Geometry: final body of the model. Coordinates: model frame, mm. Face numbers are marked on the shaded views. A direction names the side the tool comes from. Coordinates: 2 decimals unless noted, no trailing zeros. Order: outer loops, then holes, each group sorted by start corner. A loop starts at its lowest first (then second) coordinate and runs counter-clockwise, first axis right, second up. Notation, with made-up numbers: M -16,-12 L 14,-12 A29 cw 14,17 Z; hole C 39.5,-13 d11. An arc over 180 degrees is marked long. Write item = value, one per line.
from build123d import *

# Parameters (mm, degrees)
EXTRUDE006_DEPTH = 7
EXTRUDE002_DEPTH = 15


with BuildPart() as extrude006:
    # Sketch007 → Extrude006 (new body)
    with BuildSketch(Plane(origin=(0, 20, 0), x_dir=(-1, 0, 0), z_dir=(0, 1, 0))):
        Polygon((-90, 0), (-69.999121, 80.000221), (-19.999121, 80.000221), (0, 0), align=None)
    extrude(amount=EXTRUDE006_DEPTH)


with BuildPart() as fusion:
    # Sketch003 → Extrude002 (new body)
    with BuildSketch(Plane.XZ):
        Polygon((6.519191, 4.955519), (24.519191, 74.72189), (66.519191, 74.72189), (84.519191, 4.955519), align=None)
    extrude(amount=EXTRUDE002_DEPTH)


with BuildPart() as fusion_1:
    # Extrude002 placement: moved
    add(fusion.part.moved(Location((0, 26, 0))))

    # Fusion: union Extrude006
    add(extrude006.part)


solid = fusion_1.part
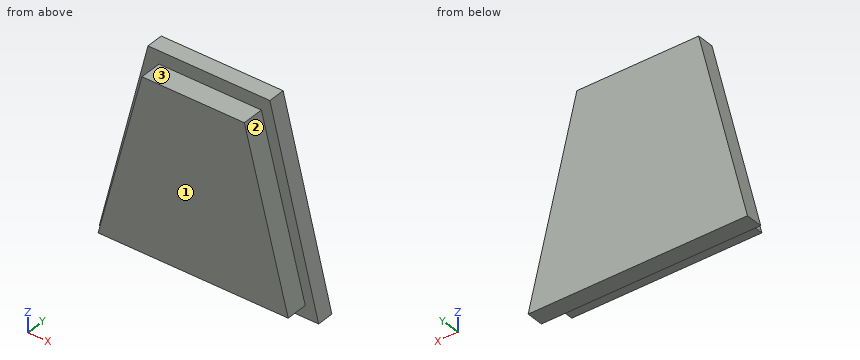
1) Section A-A, the plane x = 37.5. Return loops of the section in (y, z).
Numbers:
outline = M 11,4.96 L 20,4.96 L 20,0 L 27,0 L 27,80 L 20,80 L 20,74.72 L 11,74.72 Z
2) Line query: L1, parallel to Z at x = 26, y = 14.5; L2, parallel to Y at x = 35, z = 4; L3, parallel to X at y = 18.5, z = 68.5. Output: solid intervals per line, ascending.
Numbers:
L1 = 4.96 to 74.72
L2 = 20 to 27
L3 = 22.91 to 68.12
3) Section D-D, the plane y = 25.75. Return loops of the section in (x, z), and give its area (3 significant figures).
Numbers:
outline = M 0,0 L 90,0 L 70,80 L 20,80 Z
area = 5,600 mm²
4) Pin query (flat end, axial travel): pin 1 (7 mm diameter, centred on x = 48.5, y = 13.5, fed in from -Z); pin 2 (4 mm diameter, centred on y = 22, z = 23.5, fed in from +X). Return the tip coordinate at first contact, or that it passes through.
Numbers:
pin_1 = 4.96
pin_2 = 84.62
5) Section B-B, the plane z = 27.5. Return loops of the section in (x, y).
Numbers:
outline = M 6.87,20 L 12.34,20 L 12.34,11 L 78.7,11 L 78.7,20 L 83.12,20 L 83.12,27 L 6.87,27 Z
6) Section C-C, the plane y = 16. Return loops of the section in (x, z), and give its area (3 significant figures).
Numbers:
outline = M 6.52,4.96 L 84.52,4.96 L 66.52,74.72 L 24.52,74.72 Z
area = 4,190 mm²
7) Set-up query: the marked faces 1, 2 and 3. Return all of +Z, -Z, +X, -X, +Y, -Y with unobstructed straight access to the full face (end or side cutting, diameter ignored); none if empty.
Numbers:
face_1 = +Z, -Z, +X, -X, -Y
face_2 = +Z, +X, -Y
face_3 = +Z, +X, -X, -Y
